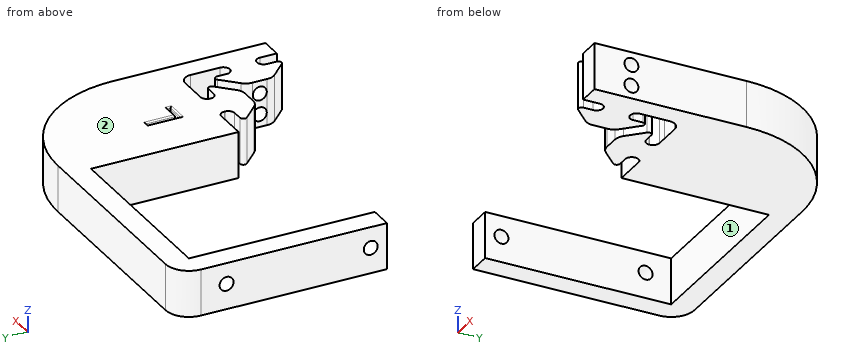
```python
from build123d import *

# Parameters (mm, degrees)
BOSS_EXTRUDE1_DEPTH = 10
CUT_EXTRUDE1_REACH  = 92.069
SKETCH2_R           = 1.5
FILLET3_R           = 5
CUT_EXTRUDE2_REACH  = 92.069
SKETCH3_R           = 1.5
FILLET4_R           = 25
CUT_EXTRUDE7_DEPTH  = 1
FILLET8_R           = 0.3
SKETCH8_W           = 10
SKETCH8_H           = 31.75
BOSS_EXTRUDE2_DEPTH = 0.8


with BuildPart() as part:
    # Sketch1 → Boss-Extrude1 (new body)
    with BuildSketch(Plane.XY):
        with BuildLine():
            Line((13.02, -7.9417418), (17.7, -7.9417418))
            Line((17.7, -7.9417418), (17.7, 49.77))
            Line((17.7, 49.77), (-56.7, 49.77))
            Line((-56.7, 49.77), (-56.7, 4.77))
            Line((-56.7, 4.77), (-51.7, 4.77))
            Line((-51.7, 4.77), (-51.7, 44.77))
            Line((-51.7, 44.77), (-10.566443095, 44.77))
            Line((-10.566443095, 44.77), (-10.566443095, 13.02))
            Line((-10.566443095, 13.02), (-5.317126718, 13.02))
            Line((-5.317126718, 13.02), (-4.287512407, 13.02))
            ThreePointArc((-4.287512407, 13.02), (-3.319474451, 12.619025549), (-2.9185, 11.650987593))
            Line((-2.9185, 11.650987593), (-2.9185, 11.539212407))
            ThreePointArc((-2.9185, 11.539212407), (-3.319474451, 10.571174451), (-4.287512407, 10.1702))
            Line((-4.287512407, 10.1702), (-6.476788598, 10.1702))
            ThreePointArc((-6.476788598, 10.1702), (-7.136510935, 9.729114651), (-6.981020848, 8.950903446))
            Line((-6.981020848, 8.950903446), (-3.672257405, 5.649701928))
            ThreePointArc((-3.672257405, 5.649701928), (-2.746830644, 5.032499411), (-1.655778399, 4.8158))
            Line((-1.655778399, 4.8158), (1.655778399, 4.8158))
            ThreePointArc((1.655778399, 4.8158), (2.746830644, 5.032499411), (3.672257405, 5.649701928))
            Line((3.672257405, 5.649701928), (6.981020848, 8.950903446))
            ThreePointArc((6.981020848, 8.950903446), (7.136510935, 9.729114651), (6.476788598, 10.1702))
            Line((6.476788598, 10.1702), (4.287512407, 10.1702))
            ThreePointArc((4.287512407, 10.1702), (3.319474451, 10.571174451), (2.9185, 11.539212407))
            Line((2.9185, 11.539212407), (2.9185, 11.650987593))
            ThreePointArc((2.9185, 11.650987593), (3.319474451, 12.619025549), (4.287512407, 13.02))
            Line((4.287512407, 13.02), (6.332886163, 13.02))
            Line((6.332886163, 13.02), (10.562594215, 13.019824354))
            ThreePointArc((10.562594215, 13.019824354), (12.303594776, 12.313982883), (13.019956614, 10.577284622))
            Line((13.019956614, 10.577284622), (13.02, 4.287469289))
            ThreePointArc((13.02, 4.287469289), (12.619025549, 3.319431332), (11.650987593, 2.918456882))
            Line((11.650987593, 2.918456882), (11.539212407, 2.918456882))
            ThreePointArc((11.539212407, 2.918456882), (10.571174451, 3.319431332), (10.1702, 4.287469289))
            Line((10.1702, 4.287469289), (10.1702, 6.402089023))
            ThreePointArc((10.1702, 6.402089023), (9.733877283, 7.055496588), (8.963146507, 6.90287605))
            Line((8.963146507, 6.90287605), (5.667020993, 3.614283579))
            ThreePointArc((5.667020993, 3.614283579), (5.046449321, 2.687255303), (4.8285, 1.593185507))
            Line((4.8285, 1.593185507), (4.8285, -1.593185507))
            ThreePointArc((4.8285, -1.593185507), (5.046449321, -2.687255303), (5.667020993, -3.614283579))
            Line((5.667020993, -3.614283579), (8.963146507, -6.90287605))
            ThreePointArc((8.963146507, -6.90287605), (9.733877283, -7.055496588), (10.1702, -6.402089023))
            Line((10.1702, -6.402089023), (10.1702, -4.287469289))
            ThreePointArc((10.1702, -4.287469289), (10.571174451, -3.319431332), (11.539212407, -2.918456882))
            Line((11.539212407, -2.918456882), (11.650987593, -2.918456882))
            ThreePointArc((11.650987593, -2.918456882), (12.619025549, -3.319431332), (13.02, -4.287469289))
            Line((13.02, -4.287469289), (13.02, -5.3170836))
            Line((13.02, -5.3170836), (13.02, -7.9417418))
        make_face()
    extrude(amount=BOSS_EXTRUDE1_DEPTH)

    # Sketch2 → Cut-Extrude1 (cut, up to next)
    with BuildSketch(Plane.ZY.offset(56.7), mode=Mode.PRIVATE) as cut_extrude1_sk1:
        with Locations((5.5, 8.27)):
            Circle(SKETCH2_R)
    cut_extrude1_tool1 = extrude(cut_extrude1_sk1.sketch, amount=-CUT_EXTRUDE1_REACH, mode=Mode.PRIVATE) & part.part
    # Sketch2 → Cut-Extrude1 (cut, up to next)
    with BuildSketch(Plane.ZY.offset(56.7), mode=Mode.PRIVATE) as cut_extrude1_sk2:
        with Locations((5.5, 39.27)):
            Circle(SKETCH2_R)
    cut_extrude1_tool2 = extrude(cut_extrude1_sk2.sketch, amount=-CUT_EXTRUDE1_REACH, mode=Mode.PRIVATE) & part.part
    add(cut_extrude1_tool1.solids().sort_by_distance((-56.7, 8.27, 5.5))[0], mode=Mode.SUBTRACT)
    add(cut_extrude1_tool2.solids().sort_by_distance((-56.7, 39.27, 5.5))[0], mode=Mode.SUBTRACT)

    # Fillet3
    fillet3_edges = [part.edges().sort_by_distance(p)[0] for p in [
        (-56.7, 49.77, 5),
    ]]
    fillet(fillet3_edges, radius=FILLET3_R)

    # Sketch3 → Cut-Extrude2 (cut, up to next)
    with BuildSketch(Plane(origin=(17.7, 0, 0), x_dir=(0, 0, -1), z_dir=(1, 0, 0)), mode=Mode.PRIVATE) as cut_extrude2_sk1:
        with Locations((-7.25, 0)):
            Circle(SKETCH3_R)
    cut_extrude2_tool1 = extrude(cut_extrude2_sk1.sketch, amount=-CUT_EXTRUDE2_REACH, mode=Mode.PRIVATE) & part.part
    # Sketch3 → Cut-Extrude2 (cut, up to next)
    with BuildSketch(Plane(origin=(17.7, 0, 0), x_dir=(0, 0, -1), z_dir=(1, 0, 0)), mode=Mode.PRIVATE) as cut_extrude2_sk2:
        with Locations(Location((-2.75, 0, 0), (0, 0, 90))):
            Circle(SKETCH3_R)
    cut_extrude2_tool2 = extrude(cut_extrude2_sk2.sketch, amount=-CUT_EXTRUDE2_REACH, mode=Mode.PRIVATE) & part.part
    add(cut_extrude2_tool1.solids().sort_by_distance((17.7, 0, 7.25))[0], mode=Mode.SUBTRACT)
    add(cut_extrude2_tool2.solids().sort_by_distance((17.7, 0, 2.75))[0], mode=Mode.SUBTRACT)

    # Fillet4
    fillet4_edges = [part.edges().sort_by_distance(p)[0] for p in [
        (17.7, 49.77, 5),
    ]]
    fillet(fillet4_edges, radius=FILLET4_R)

    # Sketch7 → Cut-Extrude7 (cut)
    with BuildSketch(Plane.XY.offset(10)):
        Polygon((-0.90100078, 19.84300121), (-0.90100078, 27.034293528), (0.113155829, 27.034293528), (0.113155829, 20.672765708), (3.524409877, 20.672765708), (3.524409877, 19.84300121), align=None)
    extrude(amount=-CUT_EXTRUDE7_DEPTH, mode=Mode.SUBTRACT)

    # Fillet8
    fillet8_edges = [part.edges().sort_by_distance(p)[0] for p in [
        (1.311704549, 19.84300121, 10),
        (-0.90100078, 23.438647369, 10),
        (-0.393922475, 27.034293528, 10),
        (0.113155829, 23.853529618, 10),
        (1.818782853, 20.672765708, 10),
        (3.524409877, 20.257883459, 10),
        (1.311704549, 19.84300121, 9),
        (-0.90100078, 23.438647369, 9),
        (-0.393922475, 27.034293528, 9),
        (0.113155829, 23.853529618, 9),
        (1.818782853, 20.672765708, 9),
        (3.524409877, 20.257883459, 9),
    ]]
    fillet(fillet8_edges, radius=FILLET8_R)

    # Sketch8 → Boss-Extrude2 (add)
    with BuildSketch(Plane.ZY.offset(10.566443095)):
        with Locations((5, 28.895)):
            Rectangle(SKETCH8_W, SKETCH8_H)
    extrude(amount=BOSS_EXTRUDE2_DEPTH)


solid = part.part
```
Read the model definition and answer for the solid it produces. Units are mm, in the model's axes. Face numbers are marked on the shaded views. A direction names the side the tool comes from. Give positions to 0.01 mm unless a question says otherwise; leave off trailing zeros. Write each loop counter-clockwise with the first axis right and the second up, starting at its lowest first coordinate (ties: lowest second). Pieces come first, ordered by that corner, then holes. Notation, with made-up numbers: (-13.5, 88.5) - (14.5, 88.5) arc R20 cw to (14.5, 99.5) - close; hole circle Ø1 at (78.5, -10). An arc over 180 degrees is marked (long way). Write item = value, one per line. Start each with the question number.
Item 1: Find the intervals of material crossed by probe 1 along X at (y, z) = (9.5, 6.75); probe 2 along X at (y, z) = (21, 0.5); probe 3 along Y at (x, z) = (-16, 8), in increasing order. Write a range as [from, to].
Item 2: Find section A-A (y = 0). Give the vertices of the cut face in (x, z).
Item 3: Each of these flat-tipped pins is pushed along its axis until it touches: P1, Ø4, axis at y = 35.5, z = 7, coming from the +X side; P2, Ø1.1, axis at x = 5, z = 4.5, coming from the +Y side; P3, Ø6, axis at x = -2.5, y = 30, coming from the -Z side; P4, Ø3, axis at x = 5, z = 6.5, coming from the -Y side. Where does it stop, or does it pass through?
Item 4: Find section D-D (y = 39.27). Give the vertices of the cut face in (x, z).
Item 5: Find section C-C (x = -10). Give the vertices of the cut face in (y, z).
Item 6: Find section B-B (y = 22.5). Give the vertices of the cut face in (x, z), then the cut area to 3 significant figures.
Item 7: A tool of negligible diameter and unlimited length cuts with its end or side. For the marked faces 1 and 2, from which of +Z, -Z, +X, -X, +Y, -Y can it reach the whole face along a straight path? Write none if from no direction.
Response:
q1.probe_1 = [-56.7, -51.7], [-7.19, 7.19], [13.02, 17.7]
q1.probe_2 = [-56.7, -51.7], [-11.37, 17.7]
q1.probe_3 = [44.77, 49.77]
q2.outline = (4.83, 0) - (17.7, 0) - (17.7, 1.25) - (4.83, 1.25) - close; (4.83, 4.25) - (17.7, 4.25) - (17.7, 5.75) - (4.83, 5.75) - close; (4.83, 8.75) - (17.7, 8.75) - (17.7, 10) - (4.83, 10) - close
q3.P1 = 16.13
q3.P2 = 46.84
q3.P3 = 0
q3.P4 = -4.45
q4.outline = (-56.7, 0) - (-51.7, 0) - (-51.7, 4) - (-56.7, 4) - close; (-56.7, 7) - (-51.7, 7) - (-51.7, 10) - (-56.7, 10) - close; (-11.37, 0) - (13.07, 0) - (13.07, 10) - (-11.37, 10) - close
q5.outline = (13.02, 0) - (49.77, 0) - (49.77, 10) - (13.02, 10) - close
q6.outline = (-56.7, 0) - (-51.7, 0) - (-51.7, 10) - (-56.7, 10) - close; (-11.37, 0) - (17.7, 0) - (17.7, 10) - (0.41, 10) arc R0.3 ccw to (0.11, 9.7) - (0.11, 9.3) arc R0.3 cw to (-0.19, 9) - (-0.6, 9) arc R0.3 cw to (-0.9, 9.3) - (-0.9, 9.7) arc R0.3 ccw to (-1.2, 10) - (-11.37, 10) - close
q6.area = 340 mm²
q7.face_1 = +Z, -Z, -Y
q7.face_2 = +Z, +X, -X, +Y, -Y
